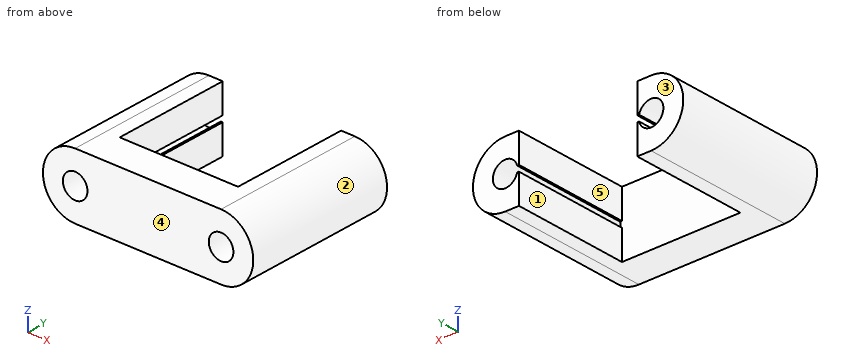
from build123d import *

# Parameters (mm, degrees)
SKETCH1_R           = 2.1
BOSS_EXTRUDE1_DEPTH = 6
BOSS_EXTRUDE2_DEPTH = 20.1


with BuildPart() as part:
    # Sketch1 → Boss-Extrude1 (new body)
    with BuildSketch(Plane(origin=(0, 0, 0), x_dir=(1, 0, 0), z_dir=(0, 1, 0))):
        with BuildLine():
            Line((0, 5.5), (24.9, 5.5))
            ThreePointArc((24.9, 5.5), (30.4, 0), (24.9, -5.5))
            Line((24.9, -5.5), (0, -5.5))
            ThreePointArc((0, -5.5), (-5.5, 0), (0, 5.5))
        make_face()
        Circle(SKETCH1_R, mode=Mode.SUBTRACT)
        with Locations((24.9, 0)):
            Circle(SKETCH1_R, mode=Mode.SUBTRACT)
    extrude(amount=BOSS_EXTRUDE1_DEPTH)

    # Sketch2 → Boss-Extrude2 (add)
    with BuildSketch(Plane(origin=(0, 6, 0), x_dir=(1, 0, 0), z_dir=(0, 1, 0))):
        with BuildLine():
            Line((22.55, 5.5), (22.55, 0.5))
            Line((22.55, 0.5), (22.860392195, 0.5))
            ThreePointArc((22.860392195, 0.5), (27, 0), (22.860392195, -0.5))
            Line((22.860392195, -0.5), (22.55, -0.5))
            Line((22.55, -0.5), (22.55, -5.5))
            Line((22.55, -5.5), (24.9, -5.5))
            ThreePointArc((24.9, -5.5), (30.4, 0), (24.9, 5.5))
            Line((24.9, 5.5), (22.55, 5.5))
        make_face()
        with BuildLine():
            Line((2.35, 5.5), (2.35, 0.5))
            Line((2.35, 0.5), (2.039607805, 0.5))
            ThreePointArc((2.039607805, 0.5), (-2.1, 0), (2.039607805, -0.5))
            Line((2.039607805, -0.5), (2.35, -0.5))
            Line((2.35, -0.5), (2.35, -5.5))
            Line((2.35, -5.5), (0, -5.5))
            ThreePointArc((0, -5.5), (-5.5, 0), (0, 5.5))
            Line((0, 5.5), (2.35, 5.5))
        make_face()
    extrude(amount=BOSS_EXTRUDE2_DEPTH)


solid = part.part
Build history of the part. All positions in model axes, mm. Face numbers are marked on the shaded views. A direction names the side the tool comes from. Coordinates: 2 decimals unless noted, no trailing zeros. Order: outer loops, then holes, each group sorted by start corner. A loop starts at its lowest first (then second) coordinate and runs counter-clockwise, first axis right, second up. Notation, with made-up numbers: (-29, 52.25) - (-21, 52.25) arc R23 ccw to (-21, 71.25) - close; hole circle Ø5 at (71.25, 28.5). An arc over 180 degrees is marked (long way). Put each result on its own line as item: value.
1. Probe line 1 along X through (y, z) = (2.55, 0); line 2 along Z through (x, y) = (0, 12); line 3 along Y through (x, z) = (12, 2). List the from-to ranges inside material, lowest first. Write a range as [from, to].
Answer sheet:
line 1: x = [-5.5, -2.1], [2.1, 22.8], [27, 30.4]
line 2: z = [-5.5, -2.1], [2.1, 5.5]
line 3: y = [0, 6]
2. Pull direction X, two halves, no side cores. Call the marked faces 1, 2 and 3: pulls with the +X half, pulls with the -X half, needs draft (parallel to the pull), parting line crosses it, or undercut.
Answer sheet:
face 1: undercut
face 2: pulls with the +X half
face 3: needs draft
3. Saw through at A-A (z = 0). Write the cut outline in (x, y), and give its area (3 significant figures).
Answer sheet:
outline: (-5.5, 0) - (-2.1, 0) - (-2.1, 26.1) - (-5.5, 26.1) - close; (2.1, 0) - (22.8, 0) - (22.8, 6) - (2.1, 6) - close; (27, 0) - (30.4, 0) - (30.4, 26.1) - (27, 26.1) - close
area: 302 mm^2
4. Saw through at D-D (z = -4.25). Write the cut outline in (x, y).
Answer sheet:
outline: (-3.49, 0) - (28.39, 0) - (28.39, 26.1) - (22.55, 26.1) - (22.55, 6) - (2.35, 6) - (2.35, 26.1) - (-3.49, 26.1) - close
5. Saw through at B-B (y = 13.5). Write the cut outline in (x, z), and give its area (3 significant figures).
Answer sheet:
outline: (0, -5.5) - (2.35, -5.5) - (2.35, -0.5) - (2.04, -0.5) arc R2.1 cw (long way) to (2.04, 0.5) - (2.35, 0.5) - (2.35, 5.5) - (0, 5.5) arc R5.5 ccw to start; (22.55, -5.5) - (24.9, -5.5) arc R5.5 ccw to (24.9, 5.5) - (22.55, 5.5) - (22.55, 0.5) - (22.86, 0.5) arc R2.1 cw (long way) to (22.86, -0.5) - (22.55, -0.5) - close
area: 118 mm^2
6. Saw through at C-C (x = 7.5). Write the cut outline in (y, z).
Answer sheet:
outline: (0, -5.5) - (6, -5.5) - (6, 5.5) - (0, 5.5) - close
7. Drop flat-ended pins along their axis: P1, Ø1.5, axis at y = 21, z = -3.5, coming from the +X side; P2, Ø5.5, axis at y = 15, z = 3, coming from the +X side; P3, Ø5.5, axis at y = 11.5, z = -3, coming from the -X side. Give the stop position or say it passes through.
Answer sheet:
P1: stops at x = 29.66
P2: stops at x = 30.39
P3: stops at x = -5.49
8. Tool access for the marked faces 4 and 5: list every direction of +Z, -Z, +X, -X, +Y, -Y with a clear straight run to the whole face (end or side of a thin tool).
Answer sheet:
face 4: +Z, -Z, +X, -X, -Y
face 5: +Z, -Z, +Y
